```python
from build123d import *

# Parameters (mm, degrees)
SKETCH_1_R      = 1.45
EXTRUDE_1_DEPTH = 2
FILLET_1_R      = 5


with BuildPart() as part:
    # 草图1 → 凸台-拉伸1 (new body)
    with BuildSketch(Plane(origin=(0, 0, 0), x_dir=(1, 0, 0), z_dir=(0, 1, 0))):
        Polygon((-17.5, -7.5), (-17.5, 7.5), (-7.5, 27.5), (7.5, 27.5), (17.5, 7.5), (17.5, -7.5), align=None)
        with Locations(Location((12.5, 0, 0), (0, 0, 270))):
            Circle(SKETCH_1_R, mode=Mode.SUBTRACT)
        with Locations(Location((0, 12.5, 0), (0, 0, 270))):
            Circle(SKETCH_1_R, mode=Mode.SUBTRACT)
        with Locations(Location((0, 22.5, 0), (0, 0, 270))):
            Circle(SKETCH_1_R, mode=Mode.SUBTRACT)
        with Locations(Location((-12.5, 0, 0), (0, 0, 90))):
            Circle(SKETCH_1_R, mode=Mode.SUBTRACT)
    extrude(amount=EXTRUDE_1_DEPTH)

    # 圆角1
    fillet_1_edges = [part.edges().sort_by_distance(p)[0] for p in [
        (17.5, 1, 7.5),
        (-17.5, 1, 7.5),
        (-17.5, 1, -7.5),
        (-7.5, 1, -27.5),
        (7.5, 1, -27.5),
        (17.5, 1, -7.5),
    ]]
    fillet(fillet_1_edges, radius=FILLET_1_R)


solid = part.part
```
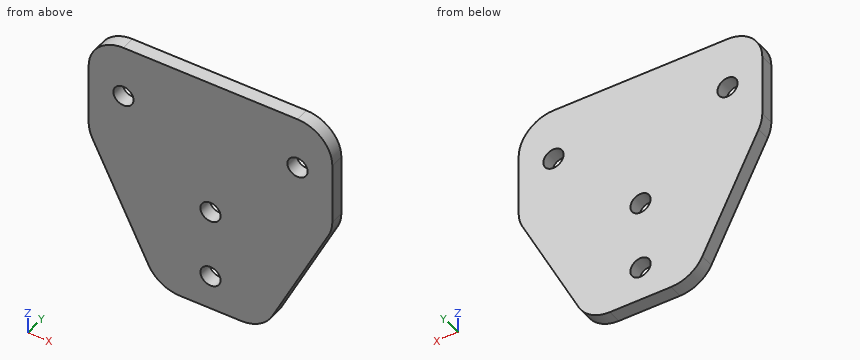
Input: part model. Units: mm. Frame: model coordinates. Give positions to 0.01 mm unless a question says otherwise; leave off trailing zeros. Write each loop counter-clockwise with the first axis right and the second up, starting at its lowest first coordinate (ties: lowest second). Pieces come first, ordered by that corner, then holes. Notation, with made-up numbers: (80, 24.5) - (116, 24.5) arc R35 cw to (116, 56.5) - close; hole circle Ø2 at (59, 73.25). An arc over 180 degrees is marked (long way). Write item = value, one per line. Start each with the question number.
1) Cut plane A-A (z = -22.5). Return loops of the section in (x, y).
2) Cut plane B-B (z = 1). Return loops of the section in (x, y).
3) Cut plane D-D (y = 1.5). Return loops of the section in (x, z), and give its area (3 significant figures).
4) Material intervals for L1, parallel to X at y = 1.55, z = 0; L2, parallel to Z at x = -12.5, y = 0.5; L3, parallel to Z at x = 1, y = 1.1, sorted ascending. Write a range as [from, to].
5) Cut plane C-C (x = 0). Return loops of the section in (y, z).
Answers follow:
q1.outline = (-10, 0) - (-1.45, 0) - (-1.45, 2) - (-10, 2) - close; (1.45, 0) - (10, 0) - (10, 2) - (1.45, 2) - close
q2.outline = (-17.5, 0) - (-13.55, 0) - (-13.55, 2) - (-17.5, 2) - close; (-11.45, 0) - (11.45, 0) - (11.45, 2) - (-11.45, 2) - close; (13.55, 0) - (17.5, 0) - (17.5, 2) - (13.55, 2) - close
q3.outline = (-17.5, -6.32) arc R5 ccw to (-16.97, -8.56) - (-8.88, -24.74) arc R5 ccw to (-4.41, -27.5) - (4.41, -27.5) arc R5 ccw to (8.88, -24.74) - (16.97, -8.56) arc R5 ccw to (17.5, -6.32) - (17.5, 2.5) arc R5 ccw to (12.5, 7.5) - (-12.5, 7.5) arc R5 ccw to (-17.5, 2.5) - close; hole circle Ø2.9 at (-12.5, 0); hole circle Ø2.9 at (0, -22.5); hole circle Ø2.9 at (0, -12.5); hole circle Ø2.9 at (12.5, 0)
q3.area = 984 mm^2
q4.L1 = [-17.5, -13.95], [-11.05, 11.05], [13.95, 17.5]
q4.L2 = [-17.5, -1.45], [1.45, 7.5]
q4.L3 = [-27.5, -23.55], [-21.45, -13.55], [-11.45, 7.5]
q5.outline = (0, -27.5) - (2, -27.5) - (2, -23.95) - (0, -23.95) - close; (0, -21.05) - (2, -21.05) - (2, -13.95) - (0, -13.95) - close; (0, -11.05) - (2, -11.05) - (2, 7.5) - (0, 7.5) - close
